Model file for the job. Use its own axes, mm. A direction names the side the tool comes from. Round coordinates to 2 decimals unless told otherwise and drop trailing zeros. Write each loop counter-clockwise with the first axis right and the second up, starting at its lowest first coordinate (ties: lowest second). Pieces come first, ordered by that corner, then holes.
```python
from build123d import *

# Parameters (mm, degrees)
ESQUISSE2_W                  = 4
ESQUISSE2_H                  = 0.5
EXTRUSION1_DEPTH             = 8.3
R_P_TITION_CIRCULAIRE1_COUNT = 2
ENL_V_MAT_EXTRU_1_DEPTH      = 131.378525839
ENL_V_MAT_EXTRU_1_DEPTH_BACK = 131.378525839
ESQUISSE3_W                  = 12
ESQUISSE3_H                  = 0.5


# Read off the part's stored shape, not the designer's step: Répétition circulaire2
with BuildPart() as part:
    # Esquisse1 → Révolution1 (revolve)
    with BuildSketch(Plane.XY, mode=Mode.PRIVATE) as r_volution1_sk:
        Polygon((0, 0), (0, 1.5), (15.7, 1.5), (15.7, 12), (17.7, 12), (17.7, 12.5), (70.2, 12.5), (70.2, 16), (108.4, 16), (108.4, 10), (111.4, 10), (111.4, 3), (128.4, 3), (128.4, 0), align=None)
    revolve(r_volution1_sk.sketch.rotate(Axis((-1000, 0, 0), (1, 0, 0)), 90), axis=Axis((-1000, 0, 0), (1, 0, 0)))

    # Esquisse2 → Extrusion1 (add)
    with BuildSketch(Plane.ZY.offset(-15.7)):
        with Locations((0, -7.8)):
            Rectangle(ESQUISSE2_W, ESQUISSE2_H)
    extrusion1 = extrude(amount=EXTRUSION1_DEPTH)

    # Répétition circulaire1: Extrusion1 ×2 about axis
    r_p_tition_circulaire1_axis = Axis((0, 0, 0), (1, 0, 0))
    for i in range(1, R_P_TITION_CIRCULAIRE1_COUNT):
        add(extrusion1.rotate(r_p_tition_circulaire1_axis, i * 360 / R_P_TITION_CIRCULAIRE1_COUNT))

    # Esquisse3 → Enlèv. mat.-Extru.1 (cut, two sides: drawn at the far end of the back side and taken through both)
    with BuildSketch(Plane.XY.offset(-ENL_V_MAT_EXTRU_1_DEPTH_BACK)):
        with Locations((122.4, 2.75)):
            Rectangle(ESQUISSE3_W, ESQUISSE3_H)
    extrude(amount=ENL_V_MAT_EXTRU_1_DEPTH + ENL_V_MAT_EXTRU_1_DEPTH_BACK, mode=Mode.SUBTRACT)

    # Esquisse5 → Trou taraudé M3x0.51 (revolve, cut)
    with BuildSketch(Plane(origin=(108.4, 13, 0), x_dir=(0, 0, -1), z_dir=(0, 1, 0))):
        Polygon((0, 0), (0, 7.251075774), (1.25, 6.5), (1.25, 0), align=None)
    revolve(axis=Axis((114.75, 13, 0), (-1, 0, 0)), mode=Mode.SUBTRACT)

    # Répétition circulaire2 outline → Répétition circulaire2 (revolve, cut)
    with BuildSketch(Plane.YX.offset(13)):
        Polygon((0, 101.148924226), (1.25, 101.9), (1.25, 108.4), (0, 108.4), align=None)
    revolve(axis=Axis((0, 0, -13), (1, 0, 0)), mode=Mode.SUBTRACT)

    # R_p_tition circulaire2 2 outline → R_p_tition circulaire2 2 (revolve, cut)
    with BuildSketch(Plane(origin=(0, -13, 0), x_dir=(0, 1, 0), z_dir=(0, 0, -1))):
        Polygon((0, 101.148924226), (1.25, 101.9), (1.25, 108.4), (0, 108.4), align=None)
    revolve(axis=Axis((0, -13, 0), (1, 0, 0)), mode=Mode.SUBTRACT)

    # R_p_tition circulaire2 3 outline → R_p_tition circulaire2 3 (revolve, cut)
    with BuildSketch(Plane.YX.offset(-13)):
        Polygon((0, 101.148924226), (1.25, 101.9), (1.25, 108.4), (0, 108.4), align=None)
    revolve(axis=Axis((0, 0, 13), (1, 0, 0)), mode=Mode.SUBTRACT)


solid = part.part
```
1) Cut at D-D on x = 74. List the corners of the cut face in (y, z).
2) Cut at B-B on y = 4.5. List the corners of the cut face in (x, z).
3) Which spindle directions (+Z, -Z, +X, -X, +Y, -Y) get a long thin tool onto all of the face, cutting with end or side? Do faces 4 (the face through (105.2, -0.16, -11.76)), 5 (the face through (70.2, 8, 10)), 6 (the face through (12, 7.55, 0)), 7 (the face through (122, 2.5, 0)), 8 (the face through (12, -8.05, 0)). Say none if no direction does.
4) Cut at C-C on x = 54.5. List the corners of the cut face in (y, z).
5) Flat gauge pins, fed straight in: pin 1 Ø10 at (x, z) = (70, 7.5) entering from +Y; pin 2 Ø3 at (x, y) = (41.5, 3.5) entering from -Z; pin 3 Ø3 at (x, z) = (11, 0) entering from +Y. Where does each tip first touch, or does it go through?
6) Cut at A-A on x = 119. List the corners of the cut face in (y, z), and give its area (3 significant figures).
7) Wall check: probe 1 along X at (y, z) = (-4, 13); probe 2 along X at (y, z) = (5.5, -6.5); probe 3 along Y at (x, z) = (51, 7.5). Give the ranges that are in metal, low to high.
8) Pull direction Z, two halves, no side cores. Call faces 1 (the face through (44.318, -3.755, 11.923)), 2 (the face through (101.279, -0.028, -12.785)), 3 (the face through (111.4, -2.4, 2.1)): released by +Z, released by -Z, zero draft, split by the parting line, or undercut.
Result sheet:
1. outline: circle Ø32 at (0, 0)
2. outline: (15.7, -11.12) - (17.7, -11.12) - (17.7, -11.66) - (70.2, -11.66) - (70.2, -15.35) - (108.4, -15.35) - (108.4, -8.93) - (111.4, -8.93) - (111.4, 8.93) - (108.4, 8.93) - (108.4, 15.35) - (70.2, 15.35) - (70.2, 11.66) - (17.7, 11.66) - (17.7, 11.12) - (15.7, 11.12) - close
3. face 4: +X
3. face 5: -X
3. face 6: +Z, -Z, -X
3. face 7: +Z, -Z, +X, +Y
3. face 8: +Z, -Z, -X, -Y
4. outline: circle Ø25 at (0, 0)
5. pin 1: stops at y = 15.8
5. pin 2: stops at z = -12.34
5. pin 3: stops at y = 8.05
6. outline: (2.5, -1.66) - (2.5, 1.66) arc R3 ccw (long way) to start
6. area: 27.1 mm2
7. probe 1: x = 70.2 to 108.4
7. probe 2: x = 15.7 to 111.4
7. probe 3: y = -10 to 10
8. face 1: split by the parting line
8. face 2: undercut
8. face 3: zero draft
